Part model, mm, in its own coordinate system. Face numbers are marked on the shaded views. A direction names the side the tool comes from. Round coordinates to 2 decimals unless told otherwise and drop trailing zeros. Write each loop counter-clockwise with the first axis right and the second up, starting at its lowest first coordinate (ties: lowest second). Pieces come first, ordered by that corner, then holes. Notation, with made-up numbers: (62.25, -30.75) -> (106.25, -30.75) arc R20 ccw to (106.25, -19.75) -> close; hole circle Ø2 at (-17.75, 82). An arc over 180 degrees is marked (long way). Use CSV: the item, a comma, the result in double quotes. Start each with the question number.
(1) Two-plate mould, pull along X, no slides. Class the marked faces 1, 2 and 3: released by +X, released by -X, zero draft, split by the parting line, or undercut.
(2) Saw through at D-D (x = -7). Give the cut face in (y, z).
(3) Drop flat-ended pins along their axis: pin 1 (1 mm diameter, centred on x = 17.5, y = 6.5, fed in from +Z); pin 2 (8 mm diameter, centred on y = -10, z = 6.5, fed in from -X); pin 3 (0.8 mm diameter, centred on x = 5, z = 8, fed in from +Y). Give the stop position or say it passes through.
(4) Saw through at A-A (x = 0). Give the cut face in (y, z).
(5) Probe line 1 (Y direction, x = 0, z = 11.25); line 2 (Z direction, x = -8, y = -14); line 3 (Y direction, x = -2.5, z = 12). List the from-to ranges inside material, lowest first. Write a range as [from, to].
(6) Which spindle directions (+Z, -Z, +X, -X, +Y, -Y) get a long thin tool onto all of the face, cutting with end or side? Do the marked faces 4 and 5. Say none if no direction does.
(7) Saw through at C-C (z = 21). Give the cut face in (x, y), plus the area to 3 significant figures.
```python
from build123d import *

# Parameters (mm, degrees)
SKETCH_1_R      = 8
SKETCH_1_R_2    = 5.1
EXTRUDE_1_DEPTH = 24
SKETCH_1_2_R    = 8
SKETCH_1_2_R_2  = 5.1
EXTRUDE_2_DEPTH = 24
SKETCH_2_R      = 22
SKETCH_2_R_2    = 8
EXTRUDE_3_DEPTH = 18
EXTRUDE_5_DEPTH = 18
EXTRUDE_6_DEPTH = 18
EXTRUDE_7_DEPTH = 18
EXTRUDE_8_DEPTH = 18


with BuildPart() as part:
    # 草图1 → 凸台-拉伸1 (new body)
    with BuildSketch(Plane.XY):
        Circle(SKETCH_1_R)
        Circle(SKETCH_1_R_2, mode=Mode.SUBTRACT)
    extrude(amount=EXTRUDE_1_DEPTH)

    # 草图1<2> → 凸台-拉伸2 (add)
    with BuildSketch(Plane.XY):
        Circle(SKETCH_1_2_R)
        Circle(SKETCH_1_2_R_2, mode=Mode.SUBTRACT)
    extrude(amount=EXTRUDE_2_DEPTH)

    # 草图2 → 凸台-拉伸3 (add)
    with BuildSketch(Plane.XY):
        Circle(SKETCH_2_R)
        Circle(SKETCH_2_R_2, mode=Mode.SUBTRACT)
    extrude(amount=EXTRUDE_3_DEPTH)

    # 草图4 → 凸台-拉伸5 (add)
    with BuildSketch(Plane.XY):
        with BuildLine():
            Line((16.379966987, 6.160087784), (20.591958498, 7.744110358))
            Line((20.591958498, 7.744110358), (20.762986314, 7.27312858))
            Line((20.762986314, 7.27312858), (20.923243358, 6.798373876))
            Line((20.923243358, 6.798373876), (21.072646499, 6.320092525))
            Line((21.072646499, 6.320092525), (21.211118232, 5.838532635))
            Line((21.211118232, 5.838532635), (16.872480412, 4.644287323))
            ThreePointArc((16.872480412, 4.644287323), (16.643489035, 5.407797402), (16.379966987, 6.160087784))
        make_face()
    extrude(amount=EXTRUDE_5_DEPTH)

    # 草图5 → 凸台-拉伸6 (add)
    with BuildSketch(Plane.XY):
        with BuildLine():
            Line((13.674702527, 10.920279795), (17.191054606, 13.728351742))
            Line((17.191054606, 13.728351742), (17.499253098, 13.333271955))
            Line((17.499253098, 13.333271955), (17.798373876, 12.93127555))
            Line((17.798373876, 12.93127555), (18.088261772, 12.522571065))
            Line((18.088261772, 12.522571065), (18.368766406, 12.107370512))
            Line((18.368766406, 12.107370512), (14.611518732, 9.630862907))
            ThreePointArc((14.611518732, 9.630862907), (14.157797402, 10.286241915), (13.674702527, 10.920279795))
        make_face()
    extrude(amount=EXTRUDE_6_DEPTH)

    # 草图6 → 凸台-拉伸7 (add)
    with BuildSketch(Plane.XY):
        with BuildLine():
            Line((9.630862907, 14.611518732), (12.107370512, 18.368766406))
            Line((12.107370512, 18.368766406), (12.522571065, 18.088261772))
            Line((12.522571065, 18.088261772), (12.93127555, 17.798373876))
            Line((12.93127555, 17.798373876), (13.333271955, 17.499253098))
            Line((13.333271955, 17.499253098), (13.728351742, 17.191054606))
            Line((13.728351742, 17.191054606), (10.920279795, 13.674702527))
            ThreePointArc((10.920279795, 13.674702527), (10.286241915, 14.157797402), (9.630862907, 14.611518732))
        make_face()
    extrude(amount=EXTRUDE_7_DEPTH)

    # 草图7 → 凸台-拉伸8 (add)
    with BuildSketch(Plane.XY):
        with BuildLine():
            Line((4.644287323, 16.872480412), (4.644287323, 21.50419948))
            Line((4.644287323, 21.50419948), (6.160087784, 21.50419948))
            Line((6.160087784, 21.50419948), (6.798373876, 20.923243358))
            Line((6.798373876, 20.923243358), (7.27312858, 20.762986314))
            Line((7.27312858, 20.762986314), (7.744110358, 20.591958498))
            Line((7.744110358, 20.591958498), (6.160087784, 16.379966987))
            ThreePointArc((6.160087784, 16.379966987), (5.407797402, 16.643489035), (4.644287323, 16.872480412))
        make_face()
    extrude(amount=EXTRUDE_8_DEPTH)


solid = part.part
```
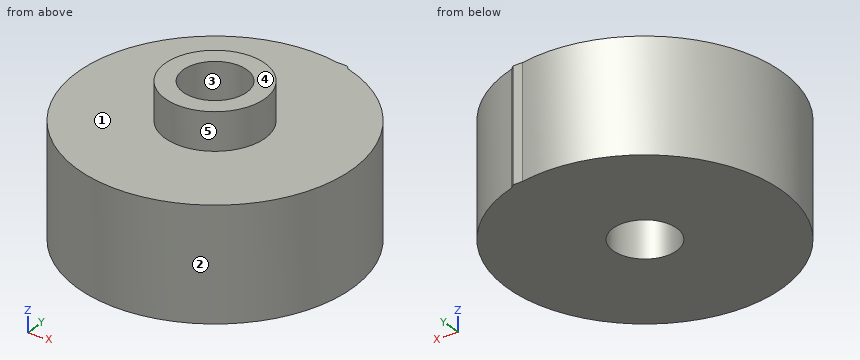
Answers:
1,face 1,"zero draft"
1,face 2,"split by the parting line"
1,face 3,"undercut"
2,outline,"(-20.86, 0) -> (20.86, 0) -> (20.86, 18) -> (3.87, 18) -> (3.87, 24) -> (-3.87, 24) -> (-3.87, 18) -> (-20.86, 18) -> close"
3,pin 1,"stops at z = 18"
3,pin 2,"stops at x = -21.17"
3,pin 3,"stops at y = 21.51"
4,outline,"(-22, 0) -> (-5.1, 0) -> (-5.1, 24) -> (-8, 24) -> (-8, 18) -> (-22, 18) -> close; (5.1, 0) -> (22, 0) -> (22, 18) -> (8, 18) -> (8, 24) -> (5.1, 24) -> close"
5,line 1,"y = [-22, -5.1], [5.1, 22]"
5,line 2,"z = [0, 18]"
5,line 3,"y = [-21.86, -4.45], [4.45, 21.86]"
6,face 4,"+Z, +X, -X, +Y, -Y"
6,face 5,"+Z"
7,outline,"circle Ø16 at (0, 0); hole circle Ø10.2 at (0, 0)"
7,area,"119 mm²"
